Read the model definition and answer for the solid it produces. Units are mm, in the model's axes. A direction names the side the tool comes from. Coordinates: 2 decimals unless noted, no trailing zeros. Order: outer loops, then holes, each group sorted by start corner. A loop starts at its lowest first (then second) coordinate and runs counter-clockwise, first axis right, second up.
```python
from build123d import *

# Parameters (mm, degrees)
BOSS_EXTRUDE1_DEPTH = 2
BOSS_EXTRUDE2_DEPTH = 6
FILLET1_R           = 2
SKETCH4_R           = 2
CUT_EXTRUDE1_DEPTH  = 50.071376586
SKETCH7_W           = 24
SKETCH7_H           = 7
CUT_EXTRUDE2_DEPTH  = 50.071376586
FILLET2_R           = 2


with BuildPart() as part:
    # Sketch1 → Boss-Extrude1 (new body)
    with BuildSketch(Plane(origin=(0, 0, 0), x_dir=(1, 0, 0), z_dir=(0, 1, 0))):
        Polygon((0, 0), (5, 0), (5, -6), (41, -6), (41, 0), (46, 0), (46, -16), (0, -16), align=None)
    extrude(amount=BOSS_EXTRUDE1_DEPTH)

    # Sketch2 → Boss-Extrude2 (add)
    with BuildSketch(Plane(origin=(0, 2, 0), x_dir=(1, 0, 0), z_dir=(0, 1, 0))):
        Polygon((0, 0), (0, -9), (46, -9), (46, 0), (41, 0), (41, -6), (5, -6), (5, 0), align=None)
    extrude(amount=BOSS_EXTRUDE2_DEPTH)

    # Fillet1
    fillet1_edges = [part.edges().sort_by_distance(p)[0] for p in [
        (46, 1, 16),
        (0, 1, 16),
        (0, 5, 9),
        (46, 5, 9),
    ]]
    fillet(fillet1_edges, radius=FILLET1_R)

    # Sketch4 → Cut-Extrude1 (cut, through all)
    with BuildSketch(Plane(origin=(0, 2, 0), x_dir=(1, 0, 0), z_dir=(0, 1, 0))):
        with Locations(Location((5, -12.8, 0), (0, 0, 270))):
            Circle(SKETCH4_R)
        with Locations(Location((41, -12.8, 0), (0, 0, 90))):
            Circle(SKETCH4_R)
    extrude(amount=-CUT_EXTRUDE1_DEPTH, mode=Mode.SUBTRACT)

    # Sketch7 → Cut-Extrude2 (cut, through all)
    with BuildSketch(Plane(origin=(0, 2, 0), x_dir=(1, 0, 0), z_dir=(0, 1, 0))):
        with Locations((23, -12.5)):
            Rectangle(SKETCH7_W, SKETCH7_H)
    extrude(amount=-CUT_EXTRUDE2_DEPTH, mode=Mode.SUBTRACT)

    # Fillet2
    fillet2_edges = [part.edges().sort_by_distance(p)[0] for p in [
        (35, 1, 16),
        (11, 1, 16),
        (11, 1, 9),
        (35, 1, 9),
    ]]
    fillet(fillet2_edges, radius=FILLET2_R)


solid = part.part
```
1) Determine the mould class of faces 1 (the flat face through (0, 3, 5)), 2 (the flat face through (41, 2, 10)), 3 (the cylindrical face through (11.6, 0.99, 9.57)), 4 (the flat face through (41, 4, 3)) for opening direction X: pulls with the +X half, pulls with the -X half, needs draft (parallel to the pull), parting line crosses it, or undercut.
A:
face 1: pulls with the -X half
face 2: needs draft
face 3: undercut
face 4: undercut
2) Which of the six approach directions +Z, -Z, +X, -X, +Y, -Y give full straight-line access (tool end or side, diameter ignored) to faces 5 (the flat face through (35, 1, 13)), 6 (the cylindrical face through (0.57, 5.04, 8.4)), 7 (the cylindrical face through (45.43, 5.04, 8.4)), 8 (the flat face through (5, 4, 3))?
A:
face 5: +Z, +Y, -Y
face 6: +Z, -X, +Y
face 7: +Z, +X, +Y
face 8: -Z, +Y, -Y
3) A cutting plane is placed at C-C, the plane z = 12.8. Determine the outline of the cut face in (x, y).
A:
outline: (0, 0) - (3, 0) - (3, 2) - (0, 2) - close; (7, 0) - (11, 0) - (11, 2) - (7, 2) - close; (35, 0) - (39, 0) - (39, 2) - (35, 2) - close; (43, 0) - (46, 0) - (46, 2) - (43, 2) - close
4) Flat-ended cylindrical pins translate along their axes: pin 1 Ø1 at (x, y) = (10.5, 5) entering from +Z; pin 2 Ø5 at (x, z) = (41, 12.8) entering from +Y. Find the tip coordinate at first contact, or state that the pin passes through.
A:
pin 1: stops at z = 9
pin 2: stops at y = 2
5) A cutting plane is placed at D-D, the plane x = 41.5. Determine the outline of the cut face in (y, z), and give its area (3 significant figures).
A:
outline: (0, 0) - (8, 0) - (8, 9) - (2, 9) - (2, 10.86) - (0, 10.86) - close; (0, 14.74) - (2, 14.74) - (2, 16) - (0, 16) - close
area: 78.3 mm2
6) A cutting plane is placed at A-A, the plane z = 1.75. Determine the outline of the cut face in (x, y), and give its area (3 significant figures).
A:
outline: (0, 0) - (5, 0) - (5, 8) - (0, 8) - close; (41, 0) - (46, 0) - (46, 8) - (41, 8) - close
area: 80.0 mm2
7) A cutting plane is placed at B-B, the plane y = 0.5. Determine the outline of the cut face in (x, z).
A:
outline: (0, 0) - (5, 0) - (5, 6) - (41, 6) - (41, 0) - (46, 0) - (46, 14) arc R2 ccw to (44, 16) - (37, 16) arc R2 ccw to (35, 14) - (35, 11) arc R2 cw to (33, 9) - (13, 9) arc R2 cw to (11, 11) - (11, 14) arc R2 ccw to (9, 16) - (2, 16) arc R2 ccw to (0, 14) - close; hole circle Ø4 at (5, 12.8); hole circle Ø4 at (41, 12.8)
8) Straight lines are drawn through the part: line 1 (X direction, y = 0.85, z = 12.8); line 2 (X direction, y = 0.75, z = 5); line 3 (Z direction, x = 29, y = 5.75). For each, find the intervals that lie inside material, in ascending order.
A:
line 1: x = 0 to 3, 7 to 11, 35 to 39, 43 to 46
line 2: x = 0 to 5, 41 to 46
line 3: z = 6 to 9
